from build123d import *

# Parameters (mm, degrees)
SKETCH1_W            = 145
SKETCH1_H            = 73
BOSS_EXTRUDE1_DEPTH  = 12.5
SKETCH2_R            = 17.5
CUT_EXTRUDE1_DEPTH   = 10
SKETCH3_W            = 5
SKETCH3_H            = 5
CUT_EXTRUDE2_DEPTH   = 10
SKETCH4_W            = 10
SKETCH4_H            = 5
BOSS_EXTRUDE2_DEPTH  = 8
SKETCH6_W            = 5
SKETCH6_H            = 73
BOSS_EXTRUDE3_DEPTH  = 15.5
SKETCH7_W            = 49
SKETCH7_H            = 36.4
CUT_EXTRUDE5_DEPTH   = 15.5
SKETCH8_W            = 29
SKETCH8_H            = 35
CUT_EXTRUDE7_DEPTH   = 10
SKETCH9_W            = 29
SKETCH9_H            = 35
BOSS_EXTRUDE4_DEPTH  = 10
SKETCH12_W           = 5
SKETCH12_H           = 1
BOSS_EXTRUDE17_DEPTH = 28
SKETCH13_W           = 5
SKETCH13_H           = 74
BOSS_EXTRUDE18_DEPTH = 1


with BuildPart() as part:
    # Sketch1 → Boss-Extrude1 (new body)
    with BuildSketch(Plane(origin=(0, 0, 0), x_dir=(1, 0, 0), z_dir=(0, 1, 0))):
        with Locations((9.033907784, -18.875048519)):
            Rectangle(SKETCH1_W, SKETCH1_H)
    extrude(amount=BOSS_EXTRUDE1_DEPTH)

    # Sketch2 → Cut-Extrude1 (cut)
    with BuildSketch(Plane(origin=(0, 12.5, 0), x_dir=(1, 0, 0), z_dir=(0, 1, 0))):
        with Locations(Location((63.533907784, -18.875048519, 0), (0, 0, 270))):
            Circle(SKETCH2_R)
    extrude(amount=-CUT_EXTRUDE1_DEPTH, mode=Mode.SUBTRACT)

    # Sketch3 → Cut-Extrude2 (cut)
    with BuildSketch(Plane(origin=(81.533907784, 0, 0), x_dir=(0, 0, -1), z_dir=(1, 0, 0))):
        with Locations((-18.721678118, 9)):
            Rectangle(SKETCH3_W, SKETCH3_H)
    extrude(amount=-CUT_EXTRUDE2_DEPTH, mode=Mode.SUBTRACT)

    # Sketch4 → Boss-Extrude2 (add)
    with BuildSketch(Plane(origin=(81.533907784, 0, 0), x_dir=(0, 0, -1), z_dir=(1, 0, 0))):
        with Locations((-18.875048519, 2.5)):
            Rectangle(SKETCH4_W, SKETCH4_H)
    extrude(amount=BOSS_EXTRUDE2_DEPTH)

    # Sketch6 → Boss-Extrude3 (add)
    with BuildSketch(Plane(origin=(0, 12.5, 0), x_dir=(1, 0, 0), z_dir=(0, 1, 0))):
        with Locations((79.033907784, -18.875048519)):
            Rectangle(SKETCH6_W, SKETCH6_H)
    extrude(amount=BOSS_EXTRUDE3_DEPTH)

    # Sketch7 → Cut-Extrude5 (cut)
    with BuildSketch(Plane(origin=(0, 12.5, 0), x_dir=(1, 0, 0), z_dir=(0, 1, 0))):
        with Locations((-38.966092216, -3.575048519)):
            Rectangle(SKETCH7_W, SKETCH7_H)
    extrude(amount=-CUT_EXTRUDE5_DEPTH, mode=Mode.SUBTRACT)

    # Sketch8 → Cut-Extrude7 (cut)
    # profile 1 of 2: a face of its own
    with BuildSketch(Plane(origin=(0, 12.5, 0), x_dir=(1, 0, 0), z_dir=(0, 1, 0))):
        with BuildLine():
            ThreePointArc((63.533907784, -36.375048519), (62.920825736, -36.364306091), (62.308496373, -36.332091994))
            Line((62.308496373, -36.332091994), (62.308496373, -43.332091994))
            Line((62.308496373, -43.332091994), (44.308496373, -43.332091994))
            Line((44.308496373, -43.332091994), (44.308496373, 13.667908006))
            Line((44.308496373, 13.667908006), (41.308496373, 13.667908006))
            Line((41.308496373, 13.667908006), (31.308496373, 13.667908006))
            Line((31.308496373, 13.667908006), (31.308496373, 10.667908006))
            Line((31.308496373, 10.667908006), (31.308496373, -43.332091994))
            Line((31.308496373, -43.332091994), (24.308496373, -43.332091994))
            Line((24.308496373, -43.332091994), (24.308496373, -27.332091994))
            Line((24.308496373, -27.332091994), (24.308496373, -24.332091994))
            Line((24.308496373, -24.332091994), (24.308496373, 13.667908006))
            Line((24.308496373, 13.667908006), (21.308496373, 13.667908006))
            Line((21.308496373, 13.667908006), (-7.691503627, 13.667908006))
            Line((-7.691503627, 13.667908006), (-10.691503627, 13.667908006))
            Line((-10.691503627, 13.667908006), (-10.691503627, 16.667908006))
            Line((-10.691503627, 16.667908006), (-13.691503627, 16.667908006))
            Line((-13.691503627, 16.667908006), (-13.691503627, 13.667908006))
            Line((-13.691503627, 13.667908006), (-13.691503627, 10.667908006))
            Line((-13.691503627, 10.667908006), (-10.691503627, 10.667908006))
            Line((-10.691503627, 10.667908006), (-10.691503627, -24.332091994))
            Line((-10.691503627, -24.332091994), (-13.691503627, -24.332091994))
            Line((-13.691503627, -24.332091994), (-13.691503627, -27.332091994))
            Line((-13.691503627, -27.332091994), (21.308496373, -27.332091994))
            Line((21.308496373, -27.332091994), (21.308496373, -43.332091994))
            Line((21.308496373, -43.332091994), (21.308496373, -46.332091994))
            Line((21.308496373, -46.332091994), (31.308496373, -46.332091994))
            Line((31.308496373, -46.332091994), (34.308496373, -46.332091994))
            Line((34.308496373, -46.332091994), (34.308496373, 10.667908006))
            Line((34.308496373, 10.667908006), (41.308496373, 10.667908006))
            Line((41.308496373, 10.667908006), (41.308496373, -43.332091994))
            Line((41.308496373, -43.332091994), (41.308496373, -46.332091994))
            Line((41.308496373, -46.332091994), (62.308496373, -46.332091994))
            Line((62.308496373, -46.332091994), (65.308496373, -46.332091994))
            Line((65.308496373, -46.332091994), (65.308496373, -36.332091994))
            Line((65.308496373, -36.332091994), (64.759319195, -36.332091994))
            ThreePointArc((64.759319195, -36.332091994), (64.146989832, -36.364306091), (63.533907784, -36.375048519))
        make_face()
        with Locations((6.808496373, -6.832091994)):
            Rectangle(SKETCH8_W, SKETCH8_H, mode=Mode.SUBTRACT)
    # profile 2 of 2: a face of its own
    with BuildSketch(Plane(origin=(0, 12.5, 0), x_dir=(1, 0, 0), z_dir=(0, 1, 0))):
        with Locations((6.808496373, -6.832091994)):
            Rectangle(SKETCH8_W, SKETCH8_H)
    extrude(amount=-CUT_EXTRUDE7_DEPTH, mode=Mode.SUBTRACT)

    # Sketch9 → Boss-Extrude4 (add)
    with BuildSketch(Plane(origin=(0, 2.5, 0), x_dir=(1, 0, 0), z_dir=(0, 1, 0))):
        with Locations((6.808496373, -6.832091994)):
            Rectangle(SKETCH9_W, SKETCH9_H)
    extrude(amount=BOSS_EXTRUDE4_DEPTH)

    # Sketch12 → Boss-Extrude17 (add)
    with BuildSketch(Plane(origin=(0, 28, 0), x_dir=(1, 0, 0), z_dir=(0, 1, 0))):
        with Locations((79.033907784, 18.124951481)):
            Rectangle(SKETCH12_W, SKETCH12_H)
    extrude(amount=-BOSS_EXTRUDE17_DEPTH)

    # Sketch13 → Boss-Extrude18 (add)
    with BuildSketch(Plane(origin=(0, 28, 0), x_dir=(1, 0, 0), z_dir=(0, 1, 0))):
        with Locations((79.033907784, -18.375048519)):
            Rectangle(SKETCH13_W, SKETCH13_H)
    extrude(amount=BOSS_EXTRUDE18_DEPTH)


solid = part.part
Input: part model. Units: mm. Frame: model coordinates. A direction names the side the tool comes from. Give positions to 0.01 mm unless a question says otherwise; leave off trailing zeros. Loops run counter-clockwise (first coordinate to the right, second up) from the corner with the lowest first, then second, coordinate; pieces in that order, holes last. Notation, with made-up numbers: (45.25, 49) -> (72.25, 49) arc R5 cw to (72.25, 53) -> close; hole circle Ø11 at (-33.5, 55). An arc over 180 degrees is marked (long way). Answer as a JSON object with one key per item and string values. Group by question number.
Item 1: Pull-direction query (Z, two-part tool) for faces 1 (the flat face through (6, 12.5, 35)), 2 (the flat face through (6, 6, -17.625)), 3 (the flat face through (78, 12.5, 19)); classes: released by +Z, released by -Z, zero draft, split by the parting line, or undercut.
Item 2: Cut plane A-A, the plane x = -22.5. Return the cut outline in (y, z).
Item 3: Cut plane C-C, the plane x = 50.5. Return the cut outline in (y, z).
Item 4: Cut plane B-B, the plane z = -1.5. Return the cut outline in (x, y), and give its area (3 significant figures).
Item 5: Pin query (flat end, axial travel): P1, Ø8, axis at y = 19.5, z = -2, coming from the +X side; P2, Ø3, axis at x = 31, y = 8, coming from the -Z side; P3, Ø8.5, axis at x = 6, z = 9, coming from the +Y side. Return the tip coordinate at first contact, or that it passes through.
Item 6: Cut plane D-D, the plane z = 39.5. Return the cut outline in (x, y), and give its area (4 significant figures).
Item 7: Reachability of faces 4 (the flat face through (-12, 8, -16.668)), 5 (the flat face through (79, 14, -18.625)), 6 (the flat face through (7, 12.5, 7)) from +Z, -Z, +X, -X, +Y, -Y: full face, straight path, thin tool, end or side. Return the list, or none.
Item 8: Line query: probe 1 along X at (y, z) = (9.5, 1); probe 2 along X at (y, z) = (10.25, 4); probe 3 along X at (y, z) = (6.5, 22). Output: solid intervals per line, ascending.
Checks:
{
 "1": {"face 1": "zero draft", "face 2": "released by -Z", "face 3": "undercut"},
 "2": {"outline": "(0, -17.62) -> (12.5, -17.62) -> (12.5, -14.62) -> (0, -14.62) -> close; (0, 21.78) -> (12.5, 21.78) -> (12.5, 55.38) -> (0, 55.38) -> close"},
 "3": {"outline": "(0, -17.62) -> (12.5, -17.62) -> (12.5, 7.2) -> (2.5, 7.2) -> (2.5, 30.55) -> (12.5, 30.55) -> (12.5, 43.33) -> (2.5, 43.33) -> (2.5, 46.33) -> (12.5, 46.33) -> (12.5, 55.38) -> (0, 55.38) -> close"},
 "4": {"outline": "(-14.47, 0) -> (81.53, 0) -> (81.53, 29) -> (76.53, 29) -> (76.53, 12.5) -> (44.31, 12.5) -> (44.31, 2.5) -> (41.31, 2.5) -> (41.31, 12.5) -> (34.31, 12.5) -> (34.31, 2.5) -> (31.31, 2.5) -> (31.31, 12.5) -> (24.31, 12.5) -> (24.31, 2.5) -> (21.31, 2.5) -> (21.31, 12.5) -> (-7.69, 12.5) -> (-7.69, 2.5) -> (-10.69, 2.5) -> (-10.69, 12.5) -> (-14.47, 12.5) -> close", "area": "1,160 mm²"},
 "5": {"P1": "stops at x = 81.53", "P2": "stops at z = -17.62", "P3": "stops at y = 12.5"},
 "6": {"outline": "(-63.47, 0) -> (81.53, 0) -> (81.53, 29) -> (76.53, 29) -> (76.53, 12.5) -> (65.31, 12.5) -> (65.31, 2.5) -> (62.31, 2.5) -> (62.31, 12.5) -> (44.31, 12.5) -> (44.31, 2.5) -> (41.31, 2.5) -> (41.31, 12.5) -> (34.31, 12.5) -> (34.31, 2.5) -> (31.31, 2.5) -> (31.31, 12.5) -> (24.31, 12.5) -> (24.31, 2.5) -> (21.31, 2.5) -> (21.31, 12.5) -> (-63.47, 12.5) -> close", "area": "1,775 mm²"},
 "7": {"face 4": "+Y", "face 5": "-Z, +X, -X, +Y, -Y", "face 6": "+Z, -Z, -X, +Y"},
 "8": {"probe 1": "x = -14.47 to -10.69, -7.69 to 21.31, 24.31 to 31.31, 34.31 to 41.31, 44.31 to 81.53", "probe 2": "x = -14.47 to -10.69, -7.69 to 21.31, 24.31 to 31.31, 34.31 to 41.31, 44.31 to 54.32, 72.75 to 81.53", "probe 3": "x = -63.47 to -10.69, -7.69 to 21.31, 24.31 to 31.31, 34.31 to 41.31, 44.31 to 46.32, 80.75 to 81.53"}
}
